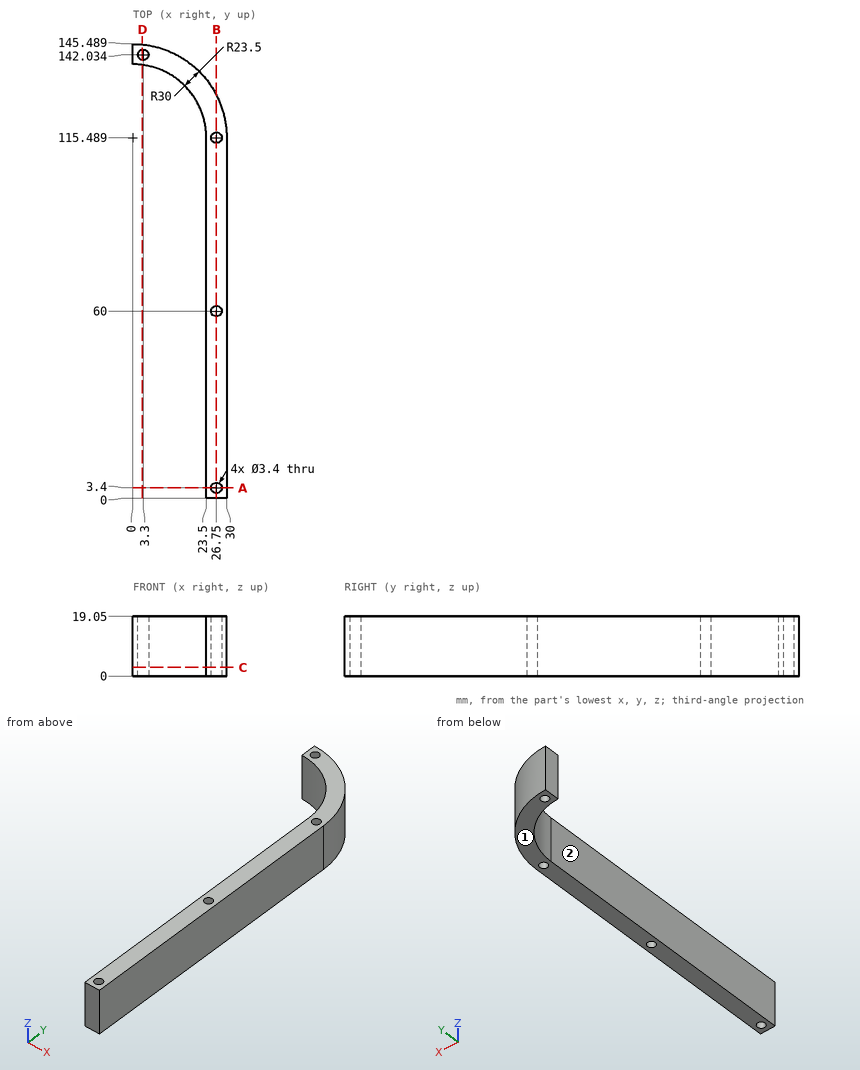
Geometry check sheet. Reference: drawing and pictorial views, mm from the part's lowest x, y, z. A direction names the side the tool comes from. Give positions to 0.01 mm unless a question says otherwise; leave off trailing zeros. Order: outer loops, then holes, each group sorted by start corner. A loop starts at its lowest first (then second) coordinate and runs counter-clockwise, first axis right, second up. Notation, with made-up numbers: M 35,2 L 47,2 A11 ccw 47,17 Z; hole C -15,-34.75 d7. An arc over 180 degrees is marked long. Answer as a JSON object with one key per item and string values. Group by question number.
1) Cross-section at D-D (x = 3). Enter the section's corners in (y, z).
2) Access from +Z, -Z, +X, -X, +Y, -Y to the whole of each face (thin tool, end or side, straight path). Record for the marked faces 1 and 2.
3) Cross-section at A-A (y = 3.4). Enter the section's corners in (x, z).
4) Scan lines: line 1 along Y through (x, z) = (26.75, 7) (1 decimal); line 2 along X through (y, z) = (55, 2.5); line 3 along Y through (x, z) = (2.5, 17.5) (1 decimal). Record each from-to range of solid material in increasing order. Write a range as [from, to].
5) Cross-section at C-C (z = 2.75). Give the number of separate pieces and of enclosed holes in the cut face.
6) Depth check by flat-ended pin: pin 1 Ø3 at (x, z) = (16.5, 15) entering from +Y; pin 2 Ø2 at (x, y) = (26.75, 60) entering from +Z; pin 3 Ø1 at (x, z) = (6, 4.5) entering from -Y; pin 4 Ø3 at (x, z) = (16.5, 2.5) entering from -Y (1 decimal). Enter the tip coordinate at first touch or a pass-through.
7) Cross-section at B-B (x = 26.75). Enter the section's corners in (y, z).
Result sheet:
{
 "1": {"outline": "M 138.8,0 L 140.36,0 L 140.36,19.05 L 138.8,19.05 Z; M 143.71,0 L 145.34,0 L 145.34,19.05 L 143.71,19.05 Z"},
 "2": {"face 1": "-Z, +X, -X, +Y, -Y", "face 2": "+Z, -Z, -X, -Y"},
 "3": {"outline": "M 23.5,0 L 25.05,0 L 25.05,19.05 L 23.5,19.05 Z; M 28.45,0 L 30,0 L 30,19.05 L 28.45,19.05 Z"},
 "4": {"line 1": "y = [0, 1.7], [5.1, 58.3], [61.7, 113.8], [117.2, 129.1]", "line 2": "x = [23.5, 30]", "line 3": "y = [138.9, 140.5], [143.5, 145.4]"},
 "5": {"separate pieces": "1", "enclosed holes": "4"},
 "6": {"pin 1": "stops at y = 141.47", "pin 2": "passes through", "pin 3": "stops at y = 138.07", "pin 4": "stops at y = 130.6"},
 "7": {"outline": "M 0,0 L 1.7,0 L 1.7,19.05 L 0,19.05 Z; M 5.1,0 L 58.3,0 L 58.3,19.05 L 5.1,19.05 Z; M 61.7,0 L 113.79,0 L 113.79,19.05 L 61.7,19.05 Z; M 117.19,0 L 129.07,0 L 129.07,19.05 L 117.19,19.05 Z"}
}
